from build123d import *

# Parameters (mm, degrees)
BOSS_EXTRUDE1_DEPTH     = 20.32
CUT_EXTRUDE1_REACH      = 45.273
SKETCH2_R               = 1.8415
CUT_EXTRUDE2_DEPTH      = 47.071427154
CUT_EXTRUDE2_DEPTH_BACK = 47.071427154
SKETCH3_R               = 1.8415


with BuildPart() as part:
    # Sketch1 → Boss-Extrude1 (new body)
    with BuildSketch(Plane(origin=(0, 0, 0), x_dir=(0, 0, -1), z_dir=(1, 0, 0))):
        Polygon((0, 8.89), (0, -8.89), (30.48, -8.89), (30.48, -13.97), (-5.08, -13.97), (-5.08, 13.97), (30.48, 13.97), (30.48, 8.89), align=None)
    extrude(amount=BOSS_EXTRUDE1_DEPTH)

    # Sketch2 → Cut-Extrude1 (cut, up to next)
    with BuildSketch(Plane.XY.offset(5.08), mode=Mode.PRIVATE) as cut_extrude1_sk1:
        with Locations((10.16, 0)):
            Circle(SKETCH2_R)
    cut_extrude1_tool1 = extrude(cut_extrude1_sk1.sketch, amount=-CUT_EXTRUDE1_REACH, mode=Mode.PRIVATE) & part.part
    add(cut_extrude1_tool1.solids().sort_by_distance((10.16, 0, 5.08))[0], mode=Mode.SUBTRACT)

    # Sketch3 → Cut-Extrude2 (cut, two sides: drawn at the far end of the back side and taken through both)
    with BuildSketch(Plane(origin=(0, 13.97, 0), x_dir=(1, 0, 0), z_dir=(0, 1, 0)).offset(-CUT_EXTRUDE2_DEPTH_BACK)):
        with Locations(Location((10.16, 8.89, 0), (0, 0, 270))):
            Circle(SKETCH3_R)
        with Locations(Location((10.16, 24.0665, 0), (0, 0, 270))):
            Circle(SKETCH3_R)
    extrude(amount=CUT_EXTRUDE2_DEPTH + CUT_EXTRUDE2_DEPTH_BACK, mode=Mode.SUBTRACT)


solid = part.part
Design review of the part built by this model. Coordinates are the model's own, in mm. A direction names the side the tool comes from. Round coordinates to 2 decimals unless told otherwise and drop trailing zeros. Order: outer loops, then holes, each group sorted by start corner. A loop starts at its lowest first (then second) coordinate and runs counter-clockwise, first axis right, second up. Notation, with made-up numbers: M 84,53.5 L 127,53.5 A21 ccw 127,67.5 Z; hole C 48,85.25 d1. An arc over 180 degrees is marked long. Answer as CSV lines item,"result". Start each with the question number.
1) The part is to be moulded in two halves that separate along Z. For faces 3 (the face through (11.9, 0.6, 2.6)), 4 (the face through (8.362, -11.466, -9.289)), 5 (the face through (10, 11, -30.48)), say which applies: +Z half, -Z half, draft (parallel to the pull), parting line (faces both ways), or undercut.
2) Tool access review of faces 1 (the face through (10, 8.89, -15)), 2 (the face through (20.32, 10, -13)): name each direction out of +Z, -Z, +X, -X, +Y, -Y from which nothing blocks a thin tool from reaching the whole face with its end or side.
3) Add section A-A (z = -8.89). Give the boundary of the cut face in (x, y).
4) For pin 1 Ø2 at (x, y) = (10.16, 0) entering from +Z; pin 2 Ø5.5 at (x, y) = (15, 1) entering from -Z, all flat-tipped, find the tip position at first contact; note any pin that passes through.
5) Add section D-D (x = 10.16). Give the boundary of the cut face in (y, z) (1 decimal), then the cut area to 3 significant figures.
6) Add section C-C (y = 0). Give the boundary of the cut face in (x, z).
7) Add section B-B (z = -15). Give the boundary of the cut face in (x, y).
8) Wall thickness on line 1 along Z through (x, y) = (10.16, 13.05) (1 decimal); line 2 along X through (y, z) = (11.3, -8.89); line 3 along Y through (x, z) = (4, -1): over which ranges is each line inside the solid? List them lowest first. Write a range as [from, to].
Resolved:
1,face 3,"draft"
1,face 4,"undercut"
1,face 5,"-Z half"
2,face 1,"-Z, +X, -X"
2,face 2,"+Z, -Z, +X, +Y, -Y"
3,outline,"M 0,-13.97 L 8.32,-13.97 L 8.32,-8.89 L 0,-8.89 Z; M 0,8.89 L 8.32,8.89 L 8.32,13.97 L 0,13.97 Z; M 12,-13.97 L 20.32,-13.97 L 20.32,-8.89 L 12,-8.89 Z; M 12,8.89 L 20.32,8.89 L 20.32,13.97 L 12,13.97 Z"
4,pin 1,"through"
4,pin 2,"z = 0"
5,outline,"M -14,-30.5 L -8.9,-30.5 L -8.9,-25.9 L -14,-25.9 Z; M -14,-22.2 L -8.9,-22.2 L -8.9,-10.7 L -14,-10.7 Z; M -14,-7 L -8.9,-7 L -8.9,0 L -1.8,0 L -1.8,5.1 L -14,5.1 Z; M 1.8,0 L 8.9,0 L 8.9,-7 L 14,-7 L 14,5.1 L 1.8,5.1 Z; M 8.9,-30.5 L 14,-30.5 L 14,-25.9 L 8.9,-25.9 Z; M 8.9,-22.2 L 14,-22.2 L 14,-10.7 L 8.9,-10.7 Z"
5,area,"358 mm^2"
6,outline,"M 0,0 L 8.32,0 L 8.32,5.08 L 0,5.08 Z; M 12,0 L 20.32,0 L 20.32,5.08 L 12,5.08 Z"
7,outline,"M 0,-13.97 L 20.32,-13.97 L 20.32,-8.89 L 0,-8.89 Z; M 0,8.89 L 20.32,8.89 L 20.32,13.97 L 0,13.97 Z"
8,line 1,"[-30.5, -25.9], [-22.2, -10.7], [-7, 5.1]"
8,line 2,"[0, 8.32], [12, 20.32]"
8,line 3,"[-13.97, -8.89], [8.89, 13.97]"
